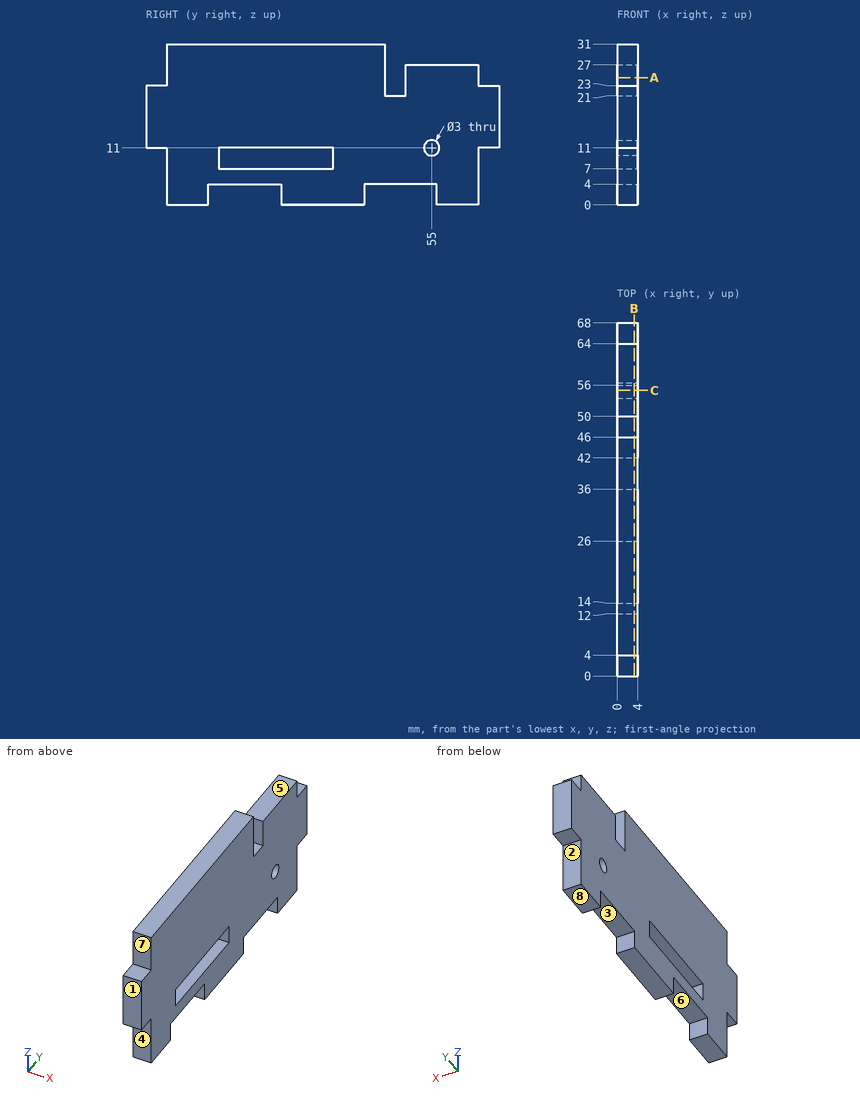
Source: three-view drawing plus pictorial views. Frame: mm from the lowest corner of the part. A direction names the side the tool comes from. Coordinates: 2 decimals unless noted, no trailing zeros. Order: outer loops, then holes, each group sorted by start corner. A loop starts at its lowest first (then second) coordinate and runs counter-clockwise, first axis right, second up.
1) Draft query along Y for the marked faces 6, 7 and 8. Return one class per face: released by +Y, released by -Y, zero draft, split by the parting line, or undercut.
Result sheet:
face 6: undercut
face 7: released by -Y
face 8: zero draft
2) Ray query, probe 1 along Z at (x, y) = (2.4, 17); probe 2 along Y at (x, z) = (2.15, 24); probe 3 along Y at (x, z) = (3.7, 22.5). Return the intervals inside material, ascending.
Result sheet:
probe 1: z = 4 to 7, 11 to 31
probe 2: y = 4 to 46, 50 to 64
probe 3: y = 0 to 46, 50 to 68
3) First-contact query: P1, Ø1.2, axis at x = 2.5, y = 24, coming from the -Z side; P2, Ø3, axis at y = 28.5, z = 20, coming from the -X side; P3, Ø1.2, axis at x = 2.5, z = 8.5, coming from the +Y side; P4, Ø1.2, axis at x = 2, y = 65.5, coming from the -Z side. Flat tips, straight axial feed; report the tip coordinate or a pass-through.
Result sheet:
P1: stops at z = 4
P2: stops at x = 0
P3: stops at y = 64
P4: stops at z = 11
4) Section B-B (x = 3.25). Give the number of separate pieces and of enclosed holes in the cut face, then the cut area to 3 significant figures.
Result sheet:
separate pieces: 1
enclosed holes: 2
area: 1,650 mm2
5) Set-up query: the marked faces 1, 2, 3, 4 and 5. Return all of +Z, -Z, +X, -X, +Y, -Y with unobstructed straight access to the full face (end or side cutting, diameter ignored); none if empty.
Result sheet:
face 1: +Z, -Z, +X, -X, -Y
face 2: -Z, +X, -X, +Y
face 3: -Z, +X, -X
face 4: -Z, +X, -X, -Y
face 5: +Z, +X, -X, +Y
6) Section C-C (y = 55). Return loops of the section in (x, z).
Result sheet:
outline: (0, 4) - (4, 4) - (4, 9.5) - (0, 9.5) - close; (0, 12.5) - (4, 12.5) - (4, 27) - (0, 27) - close
7) Section A-A (z = 24.5). Return loops of the section in (x, y).
Result sheet:
outline: (0, 4) - (4, 4) - (4, 46) - (0, 46) - close; (0, 50) - (4, 50) - (4, 64) - (0, 64) - close
